Geometry: final body of the model. Coordinates: model frame, mm. A direction names the side the tool comes from. Coordinates: 2 decimals unless noted, no trailing zeros. Write each loop counter-clockwise with the first axis right and the second up, starting at its lowest first coordinate (ties: lowest second). Pieces come first, ordered by that corner, then holes. Notation, with made-up numbers: (88.5, 82.5) -> (116.5, 82.5) arc R23 cw to (116.5, 102.5) -> close; hole circle Ø1 at (-21.75, 76.25). An arc over 180 degrees is marked (long way). One line per item, written item: value. Start each with the question number.
Autodesk Inventor part; units mm, degrees
ref_plane "YZ Plane" through (0, 0, 0) normal (1, 0, 0) x (0, 1, 0)
ref_plane "XZ Plane" through (0, 0, 0) normal (0, 1, 0) x (-1, 0, 0)
ref_plane "XY Plane" through (0, 0, 0) normal (0, 0, 1) x (1, 0, 0)
sketch "Эскиз1" plane through (0, 0, 0) normal (0, 1, 0) x (-1, 0, 0)
  circle A0 centre (0, 0) radius 45
  dimension "d0" = 90
extrude "Выдавливание1" add sketch "Эскиз1" along normal blind 15
sketch "Эскиз3" plane through (0, 0, 0) normal (0, -1, 0) x (1, 0, 0)
  circle A0 centre (0, 0) radius 30
  line L0 (-15.9099, 15.9099) -> (-21.2132, 21.2132)
  line L1 (0, 0) -> (30, 0) construction
  line L2 (-15.9099, -15.9099) -> (-21.2132, -21.2132)
  line L3 (0, 0) -> (30, 0) construction
  line L4 (15.9099, -15.9099) -> (21.2132, -21.2132)
  line L5 (0, 0) -> (30, 0) construction
  line L6 (15.9099, 15.9099) -> (21.2132, 21.2132)
  line L7 (0, 0) -> (30, 0) construction
  arc A1 (-25.812, -15.2886) -> (-15.2886, -25.812) centre (-21.2132, -21.2132) ccw
  arc A2 (-15.2886, 25.812) -> (-25.812, 15.2886) centre (-21.2132, 21.2132) ccw
  arc A3 (25.812, 15.2886) -> (15.2886, 25.812) centre (21.2132, 21.2132) ccw
  arc A4 (15.2886, -25.812) -> (25.812, -15.2886) centre (21.2132, -21.2132) ccw
  dimension "d26" = 60
  dimension "d27" = 30
  dimension "d28" = 135
  dimension "d29" = 30
  dimension "d30" = 135
  dimension "d31" = 30
  dimension "d32" = 45
  dimension "d33" = 30
  dimension "d34" = 45
  dimension "d35" = 15
  dimension "d36" = 15
  dimension "d37" = 15
  dimension "d38" = 15
extrude "Выдавливание2" add sketch "Эскиз3" along normal blind 30
sketch "Эскиз4" plane through (0, 15, 0) normal (0, 1, 0) x (1, 0, 0)
  circle A0 centre (0, 0) radius 25
  dimension "d41" = 50
extrude "Выдавливание3" add sketch "Эскиз4" along normal blind 35
sketch "Эскиз5" plane through (0, 15, 0) normal (0, 1, 0) x (1, 0, 0)
  line L0 (0, 0) -> (0, -37)
  arc A0 (15.2886, 25.812) -> (-15.2886, 25.812) centre (0, 0) ccw
  line L1 (0, 0) -> (37, 0)
  line L2 (0, 0) -> (0, 37)
  line L3 (0, 0) -> (-37, 0)
  dimension "d44" = 37
  dimension "d45" = 37
  dimension "d46" = 37
  dimension "d47" = 37
sketch "Эскиз6" plane through (0, 15, 0) normal (0, 1, 0) x (1, 0, 0)
  point P0 (37, 0)
  point P1 (0, -37)
  point P2 (-37, 0)
  point P3 (0, 37)
hole "Отверстие2" at (37, 15, 0) at (0, 15, 37) at (-37, 15, 0) at (0, 15, -37) direction (0, -1, 0) diameter 11 end through all
properties part number "КреплениеБарабана" material "Сталь, литейная"
Q1. Cut plane B-B on x = -37. Output: boundary loops of the cut face in (y, z).
Q2. First-contact query: P1, Ø2, axis at x = 24, y = 40, coming from the +Z side; P2, Ø12.5, axis at x = -37, z = 0, coming from the -Y side; P3, Ø1, axis at x = 22.5, z = 24, coming from the +Y side. Flat tips, straight axial feed; report the tip coordinate or a pass-through.
Q3. Cut plane D-D on y = -7. Output: boundary loops of the cut face in (x, z).
Q4. Draft query along X for faces 1 (the cylindrical face through (-42.453, 7.395, -0.716)), 2 (the cylindrical face through (23.846, 32.255, 7.509)), 3 (the cylindrical face through (30, -15, 0)), 4 (the flat face through (0, -30, 0)). Return one class per face: pulls with the +X half, pulls with the -X half, needs draft (parallel to the pull), parting line crosses it, or undercut.
Q5. Line query: L1, parallel to Z at x = 0, y = 7; L2, parallel to Y at x = 34, z = 20; L3, parallel to Y at x = 24.5, z = 21.5. Output: solid intervals per line, ascending. Write a range as from..to.
Q6. Access query for faces 5 (the cylindrical face through (0, -15, 30)), 6 (the cylindrical face through (0, -15, -30)), 7 (the flat face through (-9, 0, -29)), 8 (the cylindrical face through (-30, -15, 0)), 9 (the flat face through (-19, 15, -19)). Directions: +Z, -Z, +X, -X, +Y, -Y. A direction counts if a zero-diameter tool reaches every point of the face in a straight line with its end or side. Return the directions, or none.
Q7. Cut plane A-A on z = 0. Output: boundary loops of the cut face in (x, y), and give its area (3 significant figures).
Q8. Cut plane C-C on x = -3. Output: boundary loops of the cut face in (y, z).
Solution:
1. outline: (0, -25.61) -> (15, -25.61) -> (15, -5.5) -> (0, -5.5) -> close; (0, 5.5) -> (15, 5.5) -> (15, 25.61) -> (0, 25.61) -> close
2. P1: z = 9.8
2. P2: y = 0
2. P3: y = 15
3. outline: (-25.81, -15.29) arc R7.5 ccw (long way) to (-15.29, -25.81) arc R30 ccw to (15.29, -25.81) arc R7.5 ccw (long way) to (25.81, -15.29) arc R30 ccw to (25.81, 15.29) arc R7.5 ccw (long way) to (15.29, 25.81) arc R30 ccw to (-15.29, 25.81) arc R7.5 ccw (long way) to (-25.81, 15.29) arc R30 ccw to start
4. face 1: undercut
4. face 2: parting line crosses it
4. face 3: pulls with the +X half
4. face 4: needs draft
5. L1: -45..-42.5, -31.5..31.5, 42.5..45
5. L2: 0..15
5. L3: -30..15
6. face 5: +Z, -Y
6. face 6: -Z, -Y
6. face 7: -Y
6. face 8: -X, -Y
6. face 9: +Y
7. outline: (-45, 0) -> (-42.5, 0) -> (-42.5, 15) -> (-45, 15) -> close; (-31.5, 0) -> (-30, 0) -> (-30, -30) -> (30, -30) -> (30, 0) -> (31.5, 0) -> (31.5, 15) -> (25, 15) -> (25, 50) -> (-25, 50) -> (-25, 15) -> (-31.5, 15) -> close; (42.5, 0) -> (45, 0) -> (45, 15) -> (42.5, 15) -> close
7. area: 4,570 mm²
8. outline: (-30, -29.85) -> (0, -29.85) -> (0, -32.39) -> (15, -32.39) -> (15, -24.82) -> (50, -24.82) -> (50, 24.82) -> (15, 24.82) -> (15, 32.39) -> (0, 32.39) -> (0, 29.85) -> (-30, 29.85) -> close; (0, -44.9) -> (15, -44.9) -> (15, -41.61) -> (0, -41.61) -> close; (0, 41.61) -> (15, 41.61) -> (15, 44.9) -> (0, 44.9) -> close
